Job drawing, mm, ordinate dimensions from the low corner. One solid piece. A direction names the side the tool comes from. Round coordinates to 2 decimals unless told otherwise and drop trailing zeros. Loops run counter-clockwise (first coordinate to the right, second up) from the corner with the lowest first, then second, coordinate; pieces in that order, holes last. Notation, with made-up numbers: M -14,-32.75 L 45,-32.75 A31 ccw 45,2.25 Z; hole C 2,84 d9. An arc over 180 degrees is marked long. Put each result on its own line as item: value. Start each with the question number.
1) Slice it at D-D on x = 12. Give the cut face in (y, z), then the cut area to 3 significant figures.
2) Slice it at A-A on z = 3. Give the cut face in (x, y).
3) Drop flat-ended pins along their axis: pin 1 Ø2.5 at (y, z) = (17.1, 3) entering from +X; pin 2 Ø1.5 at (x, y) = (14, 7.5) entering from -Z; pin 3 Ø1 at (x, z) = (16, 3) entering from -Y; pin 4 Ø1.6 at (y, z) = (2.9, 3) entering from -X. Give the stop position or say it passes through.
4) Probe line 1 along Y through (x, z) = (1.7, 3); line 2 along X through (y, z) = (5.5, 4.15); line 3 along Y through (x, z) = (15.5, 3.1). List the from-to ranges inside material, lowest first.
5) Pull direction Z, two halves, no side cores. Call the marked faces 3, 4, 5 and 6: +Z half, -Z half, draft (parallel to the pull), parting line (faces both ways), or undercut.
6) Slice it at C-C on y = 9. Give the cut face in (x, z), then the cut area to 3 significant figures.
7) Which spindle directions (+Z, -Z, +X, -X, +Y, -Y) get a long thin tool onto all of the face, cutting with end or side? Do the marked faces 1 and 2. Say none if no direction does.
8) Slice it at B-B on x = 8.75. Give the cut face in (y, z).
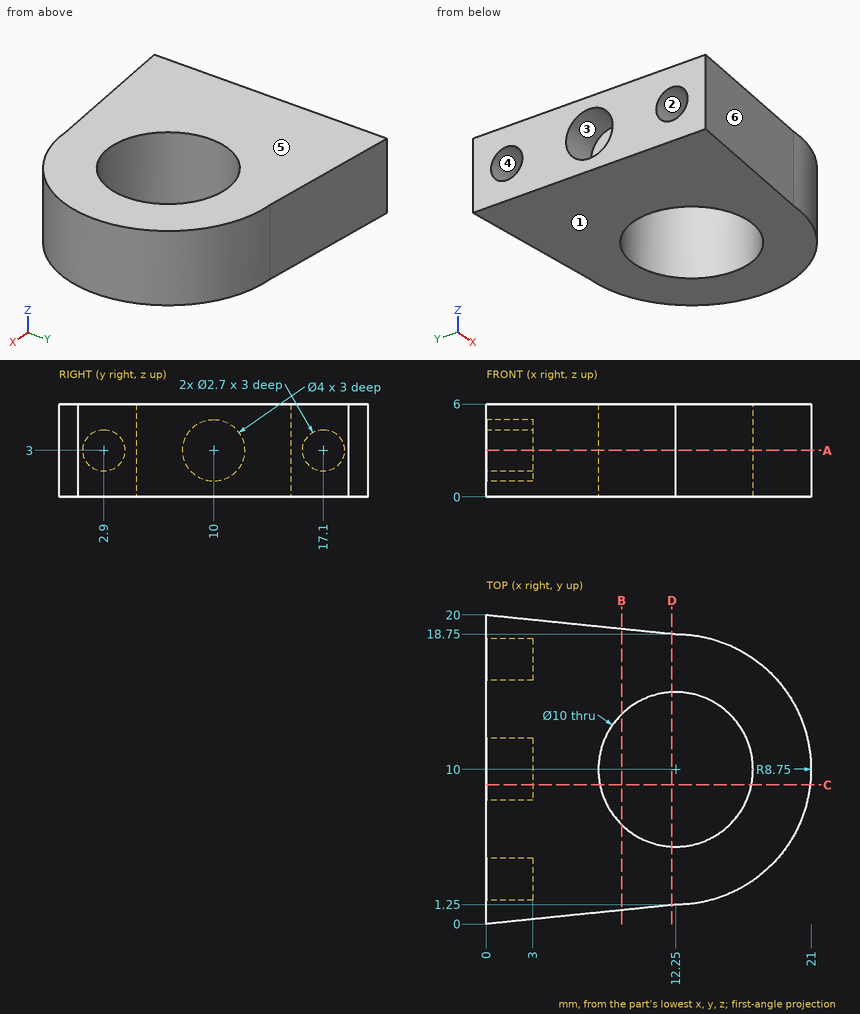
Recorded:
1. outline: M 1.22,0 L 5.01,0 L 5.01,6 L 1.22,6 Z; M 14.99,0 L 18.78,0 L 18.78,6 L 14.99,6 Z
1. area: 45.4 mm2
2. outline: M 0,0 L 12.25,1.25 A8.75 ccw 12.25,18.75 L 0,20 L 0,18.45 L 3,18.45 L 3,15.75 L 0,15.75 L 0,12 L 3,12 L 3,8 L 0,8 L 0,4.25 L 3,4.25 L 3,1.55 L 0,1.55 Z; hole C 12.25,10 d10
3. pin 1: stops at x = 18.76
3. pin 2: passes through
3. pin 3: stops at y = 1.88
3. pin 4: stops at x = 3
4. line 1: y = 0.17 to 1.55, 4.25 to 8, 12 to 15.75, 18.45 to 19.83
4. line 2: x = 0 to 10.07, 14.43 to 19.75
4. line 3: y = 1.88 to 6.2, 13.8 to 18.12
5. face 3: undercut
5. face 4: undercut
5. face 5: +Z half
5. face 6: draft
6. outline: M 0,0 L 7.35,0 L 7.35,6 L 0,6 L 0,4.73 L 3,4.73 L 3,1.27 L 0,1.27 Z; M 17.15,0 L 20.94,0 L 20.94,6 L 17.15,6 Z
6. area: 56.5 mm2
7. face 1: -Z, +X, -X, +Y, -Y
7. face 2: -X
8. outline: M 0.89,0 L 6.43,0 L 6.43,6 L 0.89,6 Z; M 13.57,0 L 19.11,0 L 19.11,6 L 13.57,6 Z
